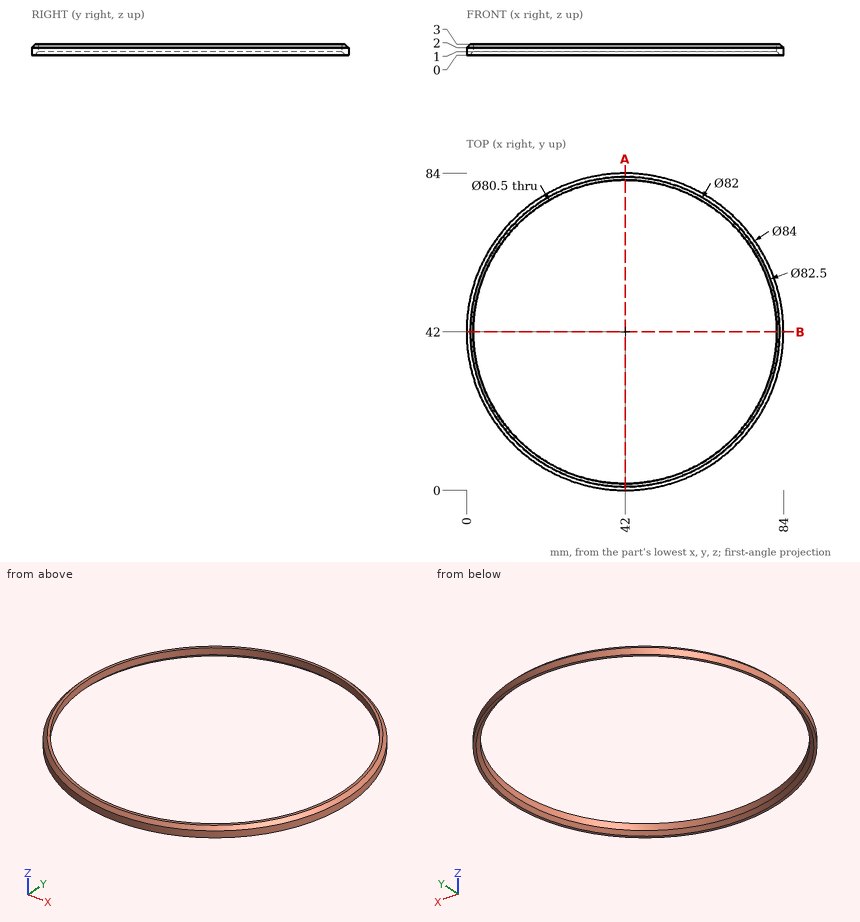
Check sheet for the drawn part. Datum: minimum x, y, z corner. Units: mm. Round coordinates to 2 decimals unless told otherwise and drop trailing zeros. Write each loop counter-clockwise with the first axis right and the second up, starting at its lowest first coordinate (ties: lowest second). Pieces come first, ordered by that corner, then holes. Notation, with made-up numbers: (35.25, 71.5) -> (62.25, 71.5) arc R14 cw to (62.25, 77.5) -> close; hole circle Ø1 at (3.5, 14). An arc over 180 degrees is marked (long way). One line per item, written item: value. Start each with the question number.
(1) Scan lines: line 1 (Y direction, x = 42, z = 1.85); line 2 (Y direction, x = 26, z = 0.45); line 3 (X direction, y = 25, z = 1.3). Record each from-to range of solid material in increasing order. Write a range as [from, to].
(2) Go/stop test with a flat-tipped pin: pin 1 Ø10 at (x, y) = (70, 67) entering from +Z. Record where the tip stops, or that it passes through.
(3) Cross-section at A-A, the plane x = 42. Record the cut outline in (y, z), and give its area (3 significant figures).
Answer:
1. line 1: [0, 1.75], [82.25, 84]
1. line 2: [3.17, 4.47], [79.53, 80.83]
1. line 3: [3.59, 5.52], [78.48, 80.41]
2. pin 1: z = 3
3. outline: (0, 0) -> (0.75, 0) -> (1.75, 1) -> (1.75, 3) -> (1, 3) -> (0, 2) -> close; (82.25, 1) -> (83.25, 0) -> (84, 0) -> (84, 2) -> (83, 3) -> (82.25, 3) -> close
3. area: 8.50 mm²
